from build123d import *

# Parameters (mm, degrees)
F2_DEPTH = 1.2
F5_DEPTH = 1.5
F7_R     = 1.1
F8_DEPTH = 1.201


with BuildPart() as f2:
    # F1 (on Top) → F2 (new body)
    with BuildSketch(Plane.XY):
        Polygon((-12.75, 17.5), (-12.75, -27.5), (12.75, -27.5), (12.75, 17.5), (33.75, 17.5), (33.75, 47.5), (-33.75, 47.5), (-33.75, 17.5), align=None)
    extrude(amount=F2_DEPTH)

    # F4 (on offset) → F5 (join)
    with BuildSketch(Plane.YZ.offset(12)):
        with BuildLine():
            Line((41.5, 4.65), (41.5, 1.2))
            Line((41.5, 1.2), (47.5, 1.2))
            Line((47.5, 1.2), (47.5, 4.65))
            ThreePointArc((47.5, 4.65), (44.5, 7.65), (41.5, 4.65))
        make_face()
    extrude(amount=F5_DEPTH)

    # F6: F2 across plane


with BuildPart() as f2_1:
    add(f2.part)
    add(f2.part.mirror(Plane.YZ))

    # F7 (on face) → F8 (cut, through all)
    with BuildSketch(Plane.XY.offset(1.2)):
        with Locations((0, 37)):
            Circle(F7_R)
        with Locations((0, 25)):
            Circle(F7_R)
        with Locations((0, -11)):
            Circle(F7_R)
        with Locations((0, -17)):
            Circle(F7_R)
    extrude(amount=-F8_DEPTH, mode=Mode.SUBTRACT)


solid = f2_1.part
Check sheet for the modelled part. Datum: model origin and axes. Units: mm. A direction names the side the tool comes from. Round coordinates to 2 decimals unless told otherwise and drop trailing zeros. Loops run counter-clockwise (first coordinate to the right, second up) from the corner with the lowest first, then second, coordinate; pieces in that order, holes last. Notation, with made-up numbers: (6, 21) -> (63, 21) arc R25 ccw to (63, 34) -> close; hole circle Ø10 at (22.5, -14.5). An arc over 180 degrees is marked (long way). Put each result on its own line as item: value. Start each with the question number.
1. Section check A-A (y = 25). Enter the section's corners in (x, z), plus the area to 3 significant figures.
2. Section check D-D (x = -16.5). Enter the section's corners in (y, z).
3. Gauge pin test, flat ends, axial feed: pin 1 (3 mm diameter, centred on y = 46, z = 4.5, fed in from +X); pin 2 (1.8 mm diameter, centred on y = 43.5, z = 4.5, fed in from -X); pin 3 (12 mm diameter, centred on x = -17, y = 24, fed in from +Z). Record the tip position at first contact, or that the pin passes through.
4. Section check B-B (x = 0). Enter the section's corners in (y, z), plus the area to 3 significant figures.
5. Section check C-C (z = 6.75). Enter the section's corners in (x, y), plus the area to 3 significant figures.
6. Draft check along X on faces 1 (the face through (0, 19, 0)), 2 (the face through (-13.5, 44, 4)), 3 (the face through (-0.238, 23.926, 0.608)), 4 (the face through (-0.14, 38.09, 0.61)). Enter one of: +X half, -X half, draft (parallel to the pull), parting line (faces both ways), or undercut.
7. Access from +Z, -Z, +X, -X, +Y, -Y to the whole of each face (thin tool, end or side, straight path). Record for faces 5 (the face through (13.5, 44, 4)), 6 (the face through (-12, 44, 4)), 7 (the face through (-0.238, -12.074, 0.608)).
8. Scan lines: probe 1 along Y at (x, z) = (0, 0.9); probe 2 along Z at (x, y) = (13.5, 25); probe 3 along X at (y, z) = (-23.5, 0.5). Record each from-to range of solid material in increasing order.
Findings:
1. outline: (-33.75, 0) -> (-1.1, 0) -> (-1.1, 1.2) -> (-33.75, 1.2) -> close; (1.1, 0) -> (33.75, 0) -> (33.75, 1.2) -> (1.1, 1.2) -> close
1. area: 78.4 mm^2
2. outline: (17.5, 0) -> (47.5, 0) -> (47.5, 1.2) -> (17.5, 1.2) -> close
3. pin 1: stops at x = 13.5
3. pin 2: stops at x = -13.5
3. pin 3: stops at z = 1.2
4. outline: (-27.5, 0) -> (-18.1, 0) -> (-18.1, 1.2) -> (-27.5, 1.2) -> close; (-15.9, 0) -> (-12.1, 0) -> (-12.1, 1.2) -> (-15.9, 1.2) -> close; (-9.9, 0) -> (23.9, 0) -> (23.9, 1.2) -> (-9.9, 1.2) -> close; (26.1, 0) -> (35.9, 0) -> (35.9, 1.2) -> (26.1, 1.2) -> close; (38.1, 0) -> (47.5, 0) -> (47.5, 1.2) -> (38.1, 1.2) -> close
4. area: 79.4 mm^2
5. outline: (-13.5, 42.36) -> (-12, 42.36) -> (-12, 46.64) -> (-13.5, 46.64) -> close; (12, 42.36) -> (13.5, 42.36) -> (13.5, 46.64) -> (12, 46.64) -> close
5. area: 12.9 mm^2
6. face 1: draft
6. face 2: -X half
6. face 3: undercut
6. face 4: undercut
7. face 5: +Z, +X, +Y, -Y
7. face 6: +Z, +Y, -Y
7. face 7: +Z, -Z
8. probe 1: y = -27.5 to -18.1, -15.9 to -12.1, -9.9 to 23.9, 26.1 to 35.9, 38.1 to 47.5
8. probe 2: z = 0 to 1.2
8. probe 3: x = -12.75 to 12.75
